from build123d import *

# Parameters (mm, degrees)
SKETCH1_R           = 7.1
BOSS_EXTRUDE1_DEPTH = 14.5
SKETCH2_R           = 0.75
BOSS_EXTRUDE2_DEPTH = 4
SKETCH3_R           = 1
CUT_EXTRUDE1_DEPTH  = 4
CUT_EXTRUDE2_START  = -4
SKETCH4_R           = 1
CUT_EXTRUDE2_DEPTH  = 4
CHAMFER1_SIZE       = 1
CHAMFER2_SIZE       = 0.5


with BuildPart() as part:
    # Sketch1 → Boss-Extrude1 (new body)
    with BuildSketch(Plane(origin=(0, 0, 0), x_dir=(1, 0, 0), z_dir=(0, 1, 0))):
        with Locations(Location((0, 0, 0), (0, 0, 90))):
            Circle(SKETCH1_R)
    extrude(amount=BOSS_EXTRUDE1_DEPTH)

    # Sketch2 → Boss-Extrude2 (add)
    with BuildSketch(Plane(origin=(0, 14.5, 0), x_dir=(1, 0, 0), z_dir=(0, 1, 0))):
        with Locations(Location((0, 0, 0), (0, 0, 270))):
            Circle(SKETCH2_R)
    extrude(amount=BOSS_EXTRUDE2_DEPTH)

    # Sketch3 → Cut-Extrude1 (cut)
    with BuildSketch(Plane.XZ):
        with Locations(Location((-4.5, 0, 0), (0, 0, 270))):
            Circle(SKETCH3_R)
        with Locations(Location((0, 4.5, 0), (0, 0, 270))):
            Circle(SKETCH3_R)
        with Locations(Location((0, -4.5, 0), (0, 0, 270))):
            Circle(SKETCH3_R)
        with Locations(Location((4.5, 0, 0), (0, 0, 270))):
            Circle(SKETCH3_R)
    extrude(amount=-CUT_EXTRUDE1_DEPTH, mode=Mode.SUBTRACT)

    # Sketch4 → Cut-Extrude2 (cut)
    with BuildSketch(Plane(origin=(0, 14.5, 0), x_dir=(1, 0, 0), z_dir=(0, 1, 0)).offset(CUT_EXTRUDE2_START)):
        with Locations(Location((-2.5, 0, 0), (0, 0, 270))):
            Circle(SKETCH4_R)
        with Locations(Location((0, 4.5, 0), (0, 0, 90))):
            Circle(SKETCH4_R)
        with Locations(Location((0, -4.5, 0), (0, 0, 90))):
            Circle(SKETCH4_R)
        with Locations(Location((2.5, 0, 0), (0, 0, 270))):
            Circle(SKETCH4_R)
    extrude(amount=CUT_EXTRUDE2_DEPTH, mode=Mode.SUBTRACT)

    # Chamfer1
    chamfer1_edges = [part.edges().sort_by_distance(p)[0] for p in [
        (0, 14.5, 7.1),
    ]]
    chamfer(chamfer1_edges, length=CHAMFER1_SIZE)

    # Chamfer2
    chamfer2_edges = [part.edges().sort_by_distance(p)[0] for p in [
        (0, 0, 7.1),
    ]]
    chamfer(chamfer2_edges, length=CHAMFER2_SIZE)


solid = part.part
Could you check a few things on this model? Use its own coordinates, in mm. A direction names the side the tool comes from. Give positions to 0.01 mm unless a question says otherwise; leave off trailing zeros. Write each loop counter-clockwise with the first axis right and the second up, starting at its lowest first coordinate (ties: lowest second). Pieces come first, ordered by that corner, then holes. Notation, with made-up numbers: (-7.75, 9) - (37.25, 9) arc R32 cw to (37.25, 47) - close; hole circle Ø2 at (-37.75, 87). An arc over 180 degrees is marked (long way). Use CSV: the item, a comma, the result in double quotes. Start each with the question number.
Item 1: I want a section at A-A, the plane x = 0. Please give me the cut outline in (y, z), then the cut area to 3 significant figures.
Item 2: I want a section at D-D, the plane y = 9.25. Please give me the cut outline in (x, z), then the cut area to 3 significant figures.
Item 3: I'm going to push flat-ended pins straight in: pin 1 (2.5 mm diameter, centred on x = 0, z = 4.5, fed in from +Y); pin 2 (1.2 mm diameter, centred on x = 0, z = 4.5, fed in from +Y); pin 3 (1.5 mm diameter, centred on y = 6.5, z = -5, fed in from +X). Where does each tip first touch, or does it pass through?
Item 4: I want a section at C-C, the plane y = 16.75. Please give me the cut outline in (x, z).
Item 5: If we mould it in two halves opening along Z, with no side actions, what happens to faces 1 (the face through (3.49, 12.47, -0.13)), 2 (the face through (0.225, 16.472, 0.715)), 3 (the face through (1, 14.5, 0))? For each: pulls with the +Z half, pulls with the -Z half, needs draft (parallel to the pull), parting line crosses it, or undercut.
Item 6: If I drill on line 1 along X through (y, z) = (12.2, 0); line 2 along X through (y, z) = (0.8, 0); line 3 along Y through (x, z) = (-2.5, -5), over which ranges is the centre line in solid material (lowest first)?
Item 7: For faces 4 (the face through (0.6, 12.5, -3.7)), 5 (the face through (-0.6, 2, -3.7)), 6 (the face through (0, 0, 0)), which set-ups out of +Z, -Z, +X, -X, +Y, -Y let a thin tool reach every point of the face, with its end or its side?
Item 8: I want a section at B-B, the plane y = 13. Please give me the cut outline in (x, z), then the cut area to 3 significant figures.
Findings:
1,outline,"(0, -6.6) - (0.5, -7.1) - (13.5, -7.1) - (14.5, -6.1) - (14.5, -5.5) - (10.5, -5.5) - (10.5, -3.5) - (14.5, -3.5) - (14.5, -0.75) - (18.5, -0.75) - (18.5, 0.75) - (14.5, 0.75) - (14.5, 3.5) - (10.5, 3.5) - (10.5, 5.5) - (14.5, 5.5) - (14.5, 6.1) - (13.5, 7.1) - (0.5, 7.1) - (0, 6.6) - (0, 5.5) - (4, 5.5) - (4, 3.5) - (0, 3.5) - (0, -3.5) - (4, -3.5) - (4, -5.5) - (0, -5.5) - close"
1,area,"179 mm2"
2,outline,"circle Ø14.2 at (0, 0)"
2,area,"158 mm2"
3,pin 1,"stops at y = 14.5"
3,pin 2,"stops at y = 10.5"
3,pin 3,"stops at x = 5.69"
4,outline,"circle Ø1.5 at (0, 0)"
5,face 1,"undercut"
5,face 2,"parting line crosses it"
5,face 3,"needs draft"
6,line 1,"x = -7.1 to -3.5, -1.5 to 1.5, 3.5 to 7.1"
6,line 2,"x = -7.1 to -5.5, -3.5 to 3.5, 5.5 to 7.1"
6,line 3,"y = 0 to 14.5"
7,face 4,"+Y"
7,face 5,"-Y"
7,face 6,"+Z, -Z, +X, -X, -Y"
8,outline,"circle Ø14.2 at (0, 0); hole circle Ø2 at (-2.5, 0); hole circle Ø2 at (0, -4.5); hole circle Ø2 at (0, 4.5); hole circle Ø2 at (2.5, 0)"
8,area,"146 mm2"
